Could you check a few things on this model? Use its own coordinates, in mm. Face numbers are marked on the shaded views. A direction names the side the tool comes from. Coordinates: 2 decimals unless noted, no trailing zeros. Order: outer loops, then holes, each group sorted by start corner. A loop starts at its lowest first (then second) coordinate and runs counter-clockwise, first axis right, second up. Notation, with made-up numbers: (-28.75, 63) -> (29.25, 63) arc R32 ccw to (29.25, 102) -> close; hole circle Ø5 at (22.5, -32). An arc over 180 degrees is marked (long way). Use a Markdown table: item, result. Add a question column.
1) If we section it at B-B (z = -355.5): Write out the boundary of the cut face in (x, y), plus the area to 3 significant figures.
2) Which directions (+Z, -Z, +X, -X, +Y, -Y) give clear straight access to the entire face, cutting with the end or side of a thin tool? Please do the marked faces 1 and 2.
3) If we section it at C-C (x = 14.5): Write out the boundary of the cut face in (y, z).
4) If we section it at A-A (z = -21): Write out the boundary of the cut face in (x, y).
5) Will these pins go through, and if not, where does the flat tip stop? pin 1 Ø8 at (x, z) = (19, 110) entering from +Y; pin 2 Ø14 at (y, z) = (213, 120) entering from +X; pin 3 Ø1.2 at (x, z) = (-1, -234.5) entering from -Y.
6) If I drill on L1, parallel to Z at x = -0.7, y = 55; L2, parallel to Z at x = -1, y = 155; L3, parallel to Y at x = -0.7, z = -300, over which ranges is the centre line in solid material (lowest first)? Write a range as [from, to].
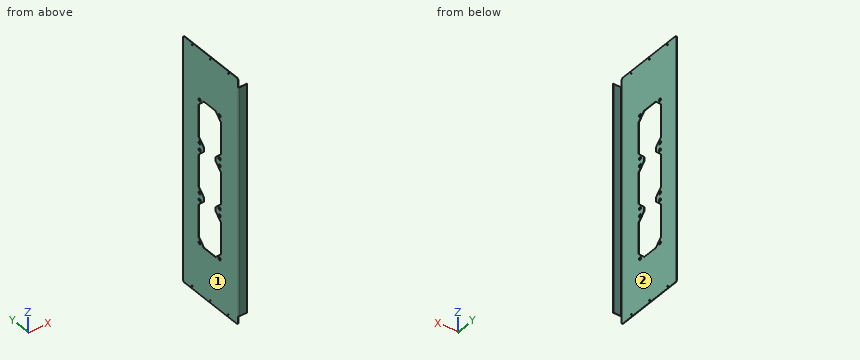
```python
from build123d import *

# Parameters (mm, degrees)
SM_BASE_FLANGE_1_DEPTH = 516
SKETCH_7_W             = 36
SKETCH_7_H             = 3
CUT_EXTRUDE_1_DEPTH    = 601.450872262
OTHER_START            = -1.5
OTHER_1_DEPTH          = 1.5
SKETCH_8_R             = 6
CUT_EXTRUDE_1446_DEPTH = 10
PATTERN_LINEAR_1_COUNT = 3
PATTERN_LINEAR_1_PITCH = 210
SKETCH_9_R             = 2.5
CUT_EXTRUDE_3_DEPTH    = 10
SKETCH_10_W            = 16
SKETCH_10_H            = 64
CUT_EXTRUDE_4_DEPTH    = 10


# Read off the part's stored shape, not the designer's step: Затупленный угол1
# Sheet-metal steps are written as plain solids
with BuildPart() as part:
    # Sketch 1 → Базовая кромка1 (new, symmetric)
    with BuildSketch(Plane.XY):
        with BuildLine():
            Line((0, 305), (0, 1.5))
            ThreePointArc((0, 1.5), (0.439339828, 0.439339828), (1.5, 0))
            Line((1.5, 0), (34, 0))
            Line((34, 0), (34, -1.5))
            Line((34, -1.5), (1.5, -1.5))
            ThreePointArc((1.5, -1.5), (-0.621320344, -0.621320344), (-1.5, 1.5))
            Line((-1.5, 1.5), (-1.5, 305))
            Line((-1.5, 305), (0, 305))
        make_face()
    extrude(amount=SM_BASE_FLANGE_1_DEPTH, both=True)

    # Эскиз7 → Вырез-Вытянуть1 (cut, through all)
    with BuildSketch(Plane.ZY.offset(1.5)):
        with Locations((-498, 0)):
            Rectangle(SKETCH_7_W, SKETCH_7_H)
        with Locations((498, 0)):
            Rectangle(SKETCH_7_W, SKETCH_7_H)
    extrude(amount=-CUT_EXTRUDE_1_DEPTH, mode=Mode.SUBTRACT)

    # Other 1 outline → Other 1 (cut)
    with BuildSketch(Plane.YZ.offset(OTHER_START)):
        Polygon((1.5, 516), (1.5, 511), (6.5, 516), align=None)
        Polygon((1.5, -516), (6.5, -516), (1.5, -511), align=None)
        Polygon((305, -516), (305, -511), (300, -516), align=None)
        Polygon((305, 516), (300, 516), (305, 511), align=None)
    extrude(amount=OTHER_1_DEPTH, mode=Mode.SUBTRACT)

    # Эскиз8 → Cut-Extrude 1446 (cut)
    with BuildSketch(Plane(origin=(0, 0, 0), x_dir=(0, 0, -1), z_dir=(1, 0, 0))):
        with Locations(Location((-300, 213, 0), (0, 0, 90))):
            Circle(SKETCH_8_R)
        with Locations(Location((-300, 103, 0), (0, 0, 90))):
            Circle(SKETCH_8_R)
        with Locations(Location((-120, 103, 0), (0, 0, 90))):
            Circle(SKETCH_8_R)
        with Locations(Location((-120, 213, 0), (0, 0, 90))):
            Circle(SKETCH_8_R)
        Polygon((-307, 126), (-277, 96), (-143, 96), (-113, 126), (-113, 190), (-143, 220), (-277, 220), (-307, 190), align=None)
    cut_extrude_1446 = extrude(amount=-CUT_EXTRUDE_1446_DEPTH, mode=Mode.SUBTRACT)

    # Линейный массив1: Cut-Extrude 1446 ×3
    with Locations(*[(0, 0, -i * PATTERN_LINEAR_1_PITCH) for i in range(1, PATTERN_LINEAR_1_COUNT)]):
        add(cut_extrude_1446, mode=Mode.SUBTRACT)

    # Эскиз9 → Вырез-Вытянуть3 (cut)
    with BuildSketch(Plane(origin=(0, 0, 0), x_dir=(0, 0, -1), z_dir=(1, 0, 0))):
        with Locations(Location((-506, 255, 0), (0, 0, 90))):
            Circle(SKETCH_9_R)
        with Locations(Location((-506, 155, 0), (0, 0, 90))):
            Circle(SKETCH_9_R)
        with Locations(Location((-506, 55, 0), (0, 0, 90))):
            Circle(SKETCH_9_R)
        with Locations(Location((506, 55, 0), (0, 0, 270))):
            Circle(SKETCH_9_R)
        with Locations(Location((506, 155, 0), (0, 0, 270))):
            Circle(SKETCH_9_R)
        with Locations(Location((506, 255, 0), (0, 0, 270))):
            Circle(SKETCH_9_R)
    extrude(amount=-CUT_EXTRUDE_3_DEPTH, mode=Mode.SUBTRACT)

    # Эскиз10 → Вырез-Вытянуть4 (cut)
    with BuildSketch(Plane(origin=(0, 0, 0), x_dir=(0, 0, -1), z_dir=(1, 0, 0))):
        with Locations((-105, 158)):
            Rectangle(SKETCH_10_W, SKETCH_10_H)
        with Locations((105, 158)):
            Rectangle(SKETCH_10_W, SKETCH_10_H)
    extrude(amount=-CUT_EXTRUDE_4_DEPTH, mode=Mode.SUBTRACT)


solid = part.part
```
Answer sheet:
| question | item | result |
|---|---|---|
| 1 | outline | (-1.5, 1.5) arc R3 ccw to (1.5, -1.5) -> (34, -1.5) -> (34, 0) -> (1.5, 0) arc R1.5 cw to (0, 1.5) -> (0, 305) -> (-1.5, 305) -> close |
| 1 | area | 509 mm2 |
| 2 | face 1 | +Z, -Z, -X, +Y, -Y |
| 2 | face 2 | +Z, -Z, +X, +Y |
| 3 | outline | (-1.5, -480) -> (0, -480) -> (0, 480) -> (-1.5, 480) -> close |
| 4 | outline | (-1.5, 1.5) arc R3 ccw to (1.5, -1.5) -> (34, -1.5) -> (34, 0) -> (1.5, 0) arc R1.5 cw to (0, 1.5) -> (0, 96) -> (-1.5, 96) -> close; (-1.5, 220) -> (0, 220) -> (0, 305) -> (-1.5, 305) -> close |
| 5 | pin 1 | y = 0 |
| 5 | pin 2 | x = 0 |
| 5 | pin 3 | y = -0.82 |
| 6 | L1 | [-516, -508.5], [-503.5, 503.5], [508.5, 516] |
| 6 | L2 | [-516, -508.5], [-503.5, -307], [307, 503.5], [508.5, 516] |
| 6 | L3 | [-0.54, 97], [109, 119], [197, 207], [219, 305] |
